Geometry: see drawing. Coordinates: mm, zero at the bounding-box minimum. Give positions to 0.01 mm unless a question says otherwise; leave off trailing zeros. Loops run counter-clockwise (first coordinate to the right, second up) from the corner with the lowest first, then second, coordinate; pieces in that order, holes last. Notation, with made-up numbers: (10.5, 85.5) -> (21.5, 85.5) arc R17 cw to (21.5, 112.5) -> close; hole circle Ø7 at (12, 74). An arc over 180 degrees is marked (long way). One line per question, with ' | ' between items.
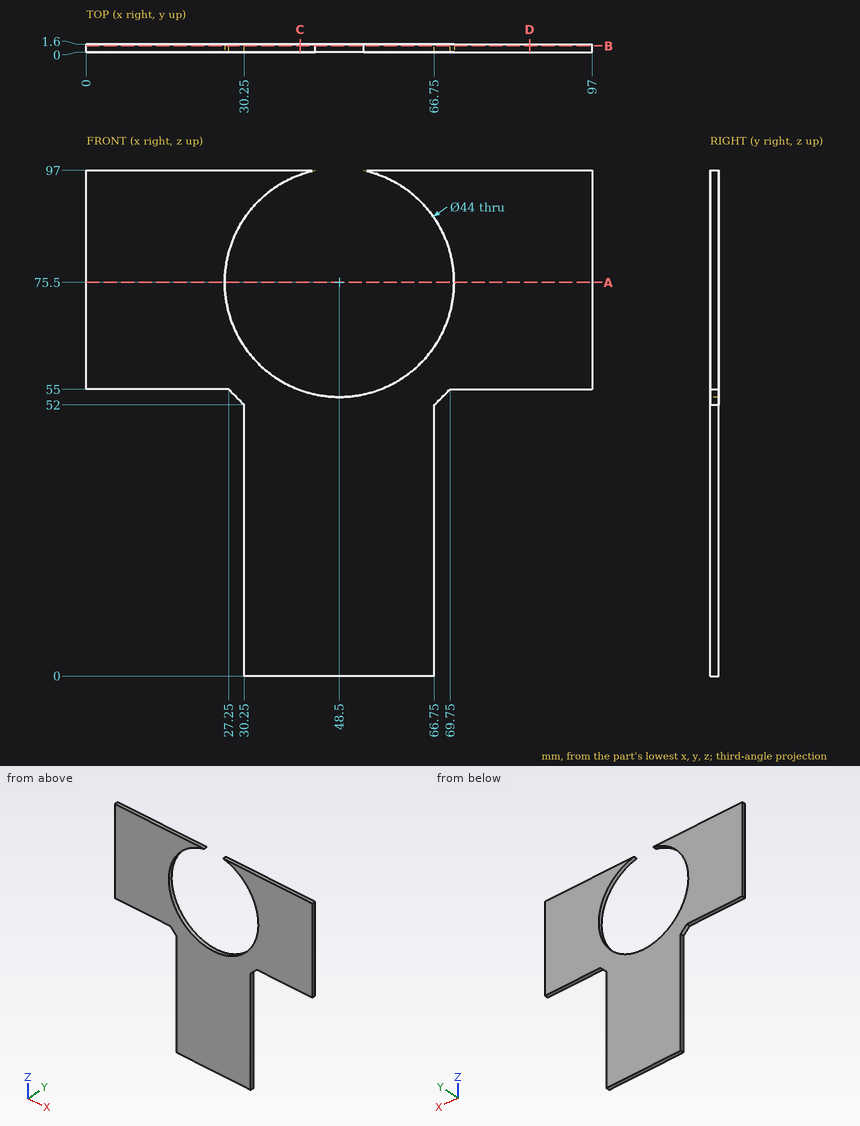
1. Ray query, line 1 along X through (y, z) = (0.7, 75.5); line 2 along X through (y, z) = (0.3, 43); line 3 along Z through (x, y) = (48.5, 1.2). Return the intervals inside material, ascending. Write a range as from..to.
Determined:
line 1: x = 0..26.5, 70.5..97 | line 2: x = 30.25..66.75 | line 3: z = 0..53.5
2. Section query D-D (x = 85). Output: boundary loops of the cut face in (y, z), then the cut area to 3 significant figures.
Determined:
outline: (0, 55) -> (1.6, 55) -> (1.6, 97) -> (0, 97) -> close | area: 67.2 mm2
3. Section query C-C (x = 41). Output: boundary loops of the cut face in (y, z), then the cut area to 3 significant figures.
Determined:
outline: (0, 0) -> (1.6, 0) -> (1.6, 54.82) -> (0, 54.82) -> close; (0, 96.18) -> (1.6, 96.18) -> (1.6, 97) -> (0, 97) -> close | area: 89.0 mm2
4. Section query A-A (z = 75.5). Output: boundary loops of the cut face in (x, y), then the cut area to 3 significant figures.
Determined:
outline: (0, 0) -> (26.5, 0) -> (26.5, 1.6) -> (0, 1.6) -> close; (70.5, 0) -> (97, 0) -> (97, 1.6) -> (70.5, 1.6) -> close | area: 84.8 mm2
5. Pin query (flat end, axial travel): P1, Ø0.5, axis at y = 0.5, z = 28.5, coming from the -X side; P2, Ø8, axis at x = 60, z = 11.5, coming from the -Y side; P3, Ø0.5, axis at x = 90, y = 1, coming from the -Z side; P4, Ø5, axis at x = 74, z = 52, coming from the -Y side. Return the tip coordinate at first contact, or that it passes through.
Determined:
P1: stops at x = 30.25 | P2: stops at y = 0 | P3: stops at z = 55 | P4: passes through
6. Section query B-B (y = 1.25). Output: boundary loops of the cut face in (x, z).
Determined:
outline: (0, 55) -> (27.25, 55) -> (30.25, 52) -> (30.25, 0) -> (66.75, 0) -> (66.75, 52) -> (69.75, 55) -> (97, 55) -> (97, 97) -> (53.16, 97) arc R22 cw (long way) to (43.84, 97) -> (0, 97) -> close
